from build123d import *

# Parameters (mm, degrees)
F0_R         = 3
F1_DEPTH     = 12.7
F2_W         = 12.7
F2_H         = 12.7
F3_DEPTH     = 3.175
F4_W         = 2.5373954162
F4_H         = 12.7
F4_W_2       = 2.54
F5_DEPTH     = 101.6
F6_T1_DEPTH  = 34.2873954162
F6_T3_DEPTH  = 34.29
F6_T8_DEPTH  = 44.45
F6_S9_R      = 3
F6_T10_DEPTH = 24
F6_T14_DEPTH = 44.45
F6_S15_R     = 3
F6_T16_DEPTH = 24
F7_W         = 3.175
F7_H         = 91.44
F8_DEPTH     = 25.4
F9_R         = 3.17499


# Not quite as in the source:
# - a fillet or chamfer that OpenCascade refuses, or shapes differently, is made with other operations: its cross-section is extruded or revolved along the edge and cut away or added
# - a fillet or chamfer is up to 0.001 mm smaller than in the source, because OpenCascade refuses the exact size


with BuildPart() as f1:
    # F0 (on Top) → F1 (new body)
    with BuildSketch(Plane.XY):
        Circle(F0_R)
    extrude(amount=F1_DEPTH)

    # F2 (on face) → F3 (join)
    with BuildSketch(Plane(origin=(0, 0, 0), x_dir=(1, 0, 0), z_dir=(0, 0, -1))):
        Rectangle(F2_W, F2_H)
    extrude(amount=F3_DEPTH)

    # F4 (on face) → F5 (join)
    with BuildSketch(Plane(origin=(0, 0, -3.175), x_dir=(1, 0, 0), z_dir=(0, 0, -1))):
        with Locations((-5.0813022919, 0)):
            Rectangle(F4_W, F4_H)
        with Locations((5.08, 0)):
            Rectangle(F4_W_2, F4_H)
    extrude(amount=F5_DEPTH)

    # F6: fillet of radius 6.35 on 6 edges, made by hand

    # F6_s2 → F6_t1 (cut)
    with BuildSketch(Plane.YZ.offset(-22.225)):
        with BuildLine():
            ThreePointArc((-6.35, -98.425), (-4.4901280605, -102.9151280605), (0, -104.775))
            Line((0, -104.775), (-6.35, -104.775))
            Line((-6.35, -104.775), (-6.35, -98.425))
        make_face()
        with BuildLine():
            ThreePointArc((6.35, -98.425), (4.4901280605, -102.9151280605), (0, -104.775))
            Line((0, -104.775), (6.35, -104.775))
            Line((6.35, -104.775), (6.35, -98.425))
        make_face()
    extrude(amount=F6_T1_DEPTH, mode=Mode.SUBTRACT)

    # F6_s4 → F6_t3 (cut)
    with BuildSketch(Plane.YZ.offset(-12.065)):
        with BuildLine():
            ThreePointArc((6.35, -98.425), (4.4901280605, -102.9151280605), (0, -104.775))
            Line((0, -104.775), (6.35, -104.775))
            Line((6.35, -104.775), (6.35, -98.425))
        make_face()
        with BuildLine():
            ThreePointArc((-6.35, -98.425), (-4.4901280605, -102.9151280605), (0, -104.775))
            Line((0, -104.775), (-6.35, -104.775))
            Line((-6.35, -104.775), (-6.35, -98.425))
        make_face()
    extrude(amount=F6_T3_DEPTH, mode=Mode.SUBTRACT)


with BuildPart() as f6_tool6:
    # F6_s7 → F6_t8 (new body)
    with BuildSketch(Plane.YZ.offset(-22.225)):
        with BuildLine():
            ThreePointArc((6.35, -6.35), (4.4901280605, -1.8598719395), (0, 0))
            Line((0, 0), (6.35, 0))
            Line((6.35, 0), (6.35, -6.35))
        make_face()
    extrude(amount=F6_T8_DEPTH)

    # F6_s9 → F6_t10 (cut, symmetric)
    with BuildSketch(Plane.XY.offset(-3.2)):
        Circle(F6_S9_R)
    extrude(amount=F6_T10_DEPTH, both=True, mode=Mode.SUBTRACT)


with BuildPart() as f1_1:
    add(f1.part)

    # F6_t5: cut F6_tool6
    add(f6_tool6.part, mode=Mode.SUBTRACT)


with BuildPart() as f6_tool12:
    # F6_s13 → F6_t14 (new body)
    with BuildSketch(Plane.YZ.offset(22.225)):
        with BuildLine():
            ThreePointArc((0, 0), (-4.4901280605, -1.8598719395), (-6.35, -6.35))
            Line((-6.35, -6.35), (-6.35, 0))
            Line((-6.35, 0), (0, 0))
        make_face()
    extrude(amount=-F6_T14_DEPTH)

    # F6_s15 → F6_t16 (cut, symmetric)
    with BuildSketch(Plane.XY.offset(-3.2)):
        Circle(F6_S15_R)
    extrude(amount=F6_T16_DEPTH, both=True, mode=Mode.SUBTRACT)


with BuildPart() as f1_2:
    add(f1_1.part)

    # F6_t11: cut F6_tool12
    add(f6_tool12.part, mode=Mode.SUBTRACT)

    # F7 (on face) → F8 (cut)
    with BuildSketch(Plane(origin=(-6.35, 0, 0), x_dir=(0, -1, 0), z_dir=(-1, 0, 0))):
        with Locations((1.5875, -52.3875)):
            Rectangle(F7_W, F7_H)
        with Locations((-1.5875, -52.3875)):
            Rectangle(F7_W, F7_H)
    extrude(amount=-F8_DEPTH, mode=Mode.SUBTRACT)

    # F9 (radius 3.175 in the source; OpenCascade refuses exactly that, so slightly less here)
    f9_edges = [f1_2.edges().sort_by_distance(p)[0] for p in [
        (-5.081302, -3.175, -98.1075),
        (-5.081302, -3.175, -6.6675),
        (-5.081302, 3.175, -6.6675),
        (5.08, 3.175, -6.6675),
        (5.08, -3.175, -6.6675),
        (-5.081302, 3.175, -98.1075),
        (5.08, 3.175, -98.1075),
        (5.08, -3.175, -98.1075),
    ]]
    fillet(f9_edges, radius=F9_R)


solid = f1_2.part
Can you work these out from the model? Positions are in its coordinate system, mm. A direction names the side the tool comes from. Coordinates: 2 decimals unless noted, no trailing zeros. Write each loop counter-clockwise with the first axis right and the second up, starting at its lowest first coordinate (ties: lowest second). Pieces come first, ordered by that corner, then holes. Notation, with made-up numbers: (-11, 80) - (25, 80) arc R17 ccw to (25, 92) - close; hole circle Ø3 at (-38.75, -5). An arc over 180 degrees is marked (long way). Return JSON: item names as keys, results as strings. Group by question number.
Item 1: If we section it at B-B (x = 0): Write out the boundary of the cut face in (y, z) (3 decimals).
Item 2: We'd pull the mould along Y, two halves only. Please class faces 1 (the face through (5, 3.175, -53)), 2 (the face through (5, -6.35, -52)), 3 (the face through (3.81, 4, -53)): pulls with the +Y half, pulls with the -Y half, needs draft (parallel to the pull), parting line crosses it, or undercut.
Item 3: Please list where these lines run through material, in increasing order: probe 1 along X at (y, z) = (-5.75, -46); probe 2 along Y at (x, z) = (5.75, -28) (3 decimals); probe 3 along Z at (x, y) = (4, 0.25).
Item 4: I'm going to push flat-ended pins straight in: pin 1 Ø5 at (x, z) = (0, -79) entering from -Y; pin 2 Ø2 at (x, y) = (-4.5, 5) entering from +Z. Where does each tip first touch, or does it pass through?
Item 5: Which directions (+Z, -Z, +X, -X, +Y, -Y) give clear straight access to the entire face, cutting with the end or side of a thin tool? Please do faces 4 (the face through (-5, -6.35, -52)), 5 (the face through (5.1, 2.27, -97.15)), 6 (the face through (0, 0, -3.175)).
Item 6: If we section it at A-A (z = -45): Write out the boundary of the cut face in (x, y) (3 decimals).
Item 7: If we section it at C-C (z = -2): Write out the boundary of the cut face in (x, y), then the cut area to 3 significant figures.
Return value:
{
 "1": {"outline": "(-5.499, -3.175) - (5.499, -3.175) arc R6.35 ccw to (3, -0.753) - (3, 12.7) - (-3, 12.7) - (-3, -0.753) arc R6.35 ccw to start"},
 "2": {"face 1": "undercut", "face 2": "pulls with the -Y half", "face 3": "needs draft"},
 "3": {"probe 1": "x = -6.35 to -3.81, 3.81 to 6.35", "probe 2": "y = -6.35 to -3.175, 3.175 to 6.35", "probe 3": "z = -104.77 to -98.1, -6.68 to 0"},
 "4": {"pin 1": "passes through", "pin 2": "stops at z = -1.42"},
 "5": {"face 4": "+Z, -Z, +X, -X, -Y", "face 5": "+X, -X", "face 6": "-Z, +Y, -Y"},
 "6": {"outline": "(-6.35, -6.35) - (-3.813, -6.35) - (-3.813, -3.175) - (-6.35, -3.175) - close; (-6.35, 3.175) - (-3.813, 3.175) - (-3.813, 6.35) - (-6.35, 6.35) - close; (3.81, -6.35) - (6.35, -6.35) - (6.35, -3.175) - (3.81, -3.175) - close; (3.81, 3.175) - (6.35, 3.175) - (6.35, 6.35) - (3.81, 6.35) - close"},
 "7": {"outline": "(-6.35, -4.63) - (6.35, -4.63) - (6.35, 4.63) - (-6.35, 4.63) - close", "area": "118 mm^2"}
}
